```python
from build123d import *

# Parameters (mm, degrees)
RESSALTO_EXTRUS_O1_DEPTH = 3
ESBO_O3_W                = 5
ESBO_O3_H                = 5.322149945
CORTE_EXTRUS_O2_DEPTH    = 4


with BuildPart() as part:
    # Esboço1 → Ressalto-extrusão1 (new body)
    with BuildSketch(Plane.XY):
        with BuildLine():
            Line((-7.94118013, 1.369756817), (-2.94118013, 1.369756817))
            Line((-2.94118013, 1.369756817), (-2.94118013, 16.369756817))
            ThreePointArc((-2.94118013, 16.369756817), (-4.405646224, 19.905290723), (-7.94118013, 21.369756817))
            Line((-7.94118013, 21.369756817), (-52.94118013, 21.369756817))
            ThreePointArc((-52.94118013, 21.369756817), (-56.476714036, 19.905290723), (-57.94118013, 16.369756817))
            Line((-57.94118013, 16.369756817), (-57.94118013, 1.369756817))
            Line((-57.94118013, 1.369756817), (-32.94118013, 1.369756817))
            Line((-32.94118013, 1.369756817), (-32.94118013, -3.630243183))
            Line((-32.94118013, -3.630243183), (-7.94118013, -3.630243183))
            Line((-7.94118013, -3.630243183), (-7.94118013, 1.369756817))
        make_face()
    extrude(amount=RESSALTO_EXTRUS_O1_DEPTH)

    # Esboço3 → Corte-extrusão2 (cut, through all)
    with BuildSketch(Plane.XY.offset(3)):
        with Locations((-37.44118013, 4.03083179)):
            Rectangle(ESBO_O3_W, ESBO_O3_H)
    extrude(amount=-CORTE_EXTRUS_O2_DEPTH, mode=Mode.SUBTRACT)


solid = part.part
```
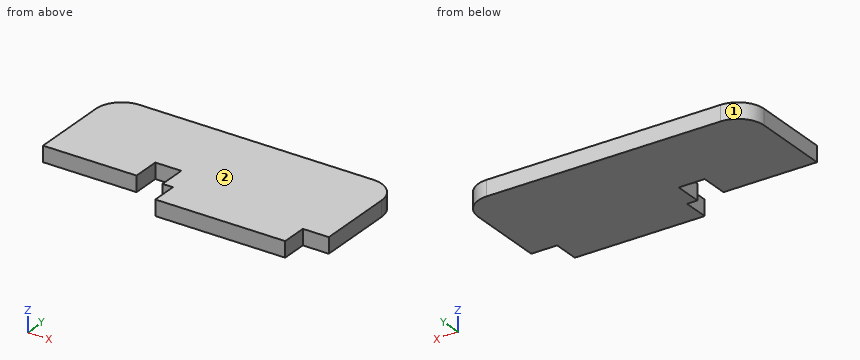
Geometry check sheet. Reference: the model listing, model coordinates, mm. Face numbers are marked on the shaded views. Coordinates: 2 decimals unless noted, no trailing zeros. Write each loop counter-clockwise with the first axis right and the second up, starting at its lowest first coordinate (ties: lowest second). Pieces come first, ordered by that corner, then holes. Notation, with made-up numbers: M 68.5,36 L 122.5,36 A4 ccw 122.5,42 Z; hole C -26.5,12 d2. An arc over 180 degrees is marked long. One line per item, written item: value. Start each with the question number.
(1) Sectioned sample at B-B, the plane y = -2. Enter the section's corners in (x, z).
(2) Sectioned sample at C-C, the plane x = -42.5. Enter the section's corners in (y, z).
(3) Depth check by flat-ended pin: pin 1 (6 mm diameter, centred on x = -37, y = 7, fed in from -Z); pin 2 (1 mm diameter, centred on x = -33.5, z = 1.5, fed in from -Y). Enter the tip coordinate at first touch or a pass-through.
(4) Release check for a two-part mould opening along X. For the marked faces 1 and 2 record: released by +X, released by -X, zero draft, split by the parting line, or undercut.
(5) Scan lines: line 1 along Y through (x, z) = (-36, 0.3); line 2 along X through (y, z) = (5.75, 1.1); line 3 along Y through (x, z) = (-42.5, 2.8). Record each from-to range of solid material in increasing order. Write a range as [from, to].
(6) Sectioned sample at A-A, the plane z = 2.05. Enter the section's corners in (x, y).
Filled sheet:
1. outline: M -32.94,0 L -7.94,0 L -7.94,3 L -32.94,3 Z
2. outline: M 1.37,0 L 21.37,0 L 21.37,3 L 1.37,3 Z
3. pin 1: z = 0
3. pin 2: y = 1.37
4. face 1: released by -X
4. face 2: zero draft
5. line 1: [6.69, 21.37]
5. line 2: [-57.94, -39.94], [-34.94, -2.94]
5. line 3: [1.37, 21.37]
6. outline: M -57.94,1.37 L -39.94,1.37 L -39.94,6.69 L -34.94,6.69 L -34.94,1.37 L -32.94,1.37 L -32.94,-3.63 L -7.94,-3.63 L -7.94,1.37 L -2.94,1.37 L -2.94,16.37 A5 ccw -7.94,21.37 L -52.94,21.37 A5 ccw -57.94,16.37 Z
